from build123d import *

# Parameters (mm, degrees)
FILLET1_R           = 5
BOSS_EXTRUDE1_DEPTH = 10
CIRPATTERN1_COUNT   = 12
SKETCH3_R           = 5
CUT_EXTRUDE1_DEPTH  = 14
FILLET2_R           = 0.5
FILLET3_R           = 0.5


with BuildPart() as part:
    # Sketch1 → Revolve1 (revolve)
    with BuildSketch(Plane(origin=(0, 0, 0), x_dir=(0, 0, -1), z_dir=(1, 0, 0))):
        Polygon((-8, 0), (8, 0), (8, -25), (-11, -25), (-11, -16), (5, -16), (5, -3), (-8, -3), align=None)
    revolve(axis=Axis((0, -25, -8), (0, 0, 1)))

    # Fillet1
    fillet1_edges = [part.edges().sort_by_distance(p)[0] for p in [
        (0, -50, -8),
    ]]
    fillet(fillet1_edges, radius=FILLET1_R)

    # Sketch2 → Boss-Extrude1 (add)
    with BuildSketch(Plane(origin=(0, 0, -8), x_dir=(-1, 0, 0), z_dir=(0, 0, -1))):
        with BuildLine():
            Line((-1, -3.05572809), (1, -3.05572809))
            Line((1, -3.05572809), (1, -16.05572809))
            ThreePointArc((1, -16.05572809), (0, -16), (-1, -16.05572809))
            Line((-1, -16.05572809), (-1, -3.05572809))
        make_face()
    boss_extrude1 = extrude(amount=-BOSS_EXTRUDE1_DEPTH)

    # CirPattern1: Boss-Extrude1 ×12 about axis
    cirpattern1_axis = Axis((0, -25, 0), (0, 0, 1))
    for i in range(1, CIRPATTERN1_COUNT):
        add(boss_extrude1.rotate(cirpattern1_axis, i * 360 / CIRPATTERN1_COUNT))

    # Sketch3 → Cut-Extrude1 (cut)
    with BuildSketch(Plane.XY.offset(11)):
        with Locations((0, -25)):
            Circle(SKETCH3_R)
    extrude(amount=-CUT_EXTRUDE1_DEPTH, mode=Mode.SUBTRACT)

    # Fillet2
    fillet2_edges = [part.edges().sort_by_distance(p)[0] for p in [
        (-5, -25, 11),
        (0, -34, 11),
    ]]
    fillet(fillet2_edges, radius=FILLET2_R)

    # Fillet3
    fillet3_edges = [part.edges().sort_by_distance(p)[0] for p in [
        (0, -50, 8),
    ]]
    fillet(fillet3_edges, radius=FILLET3_R)


solid = part.part
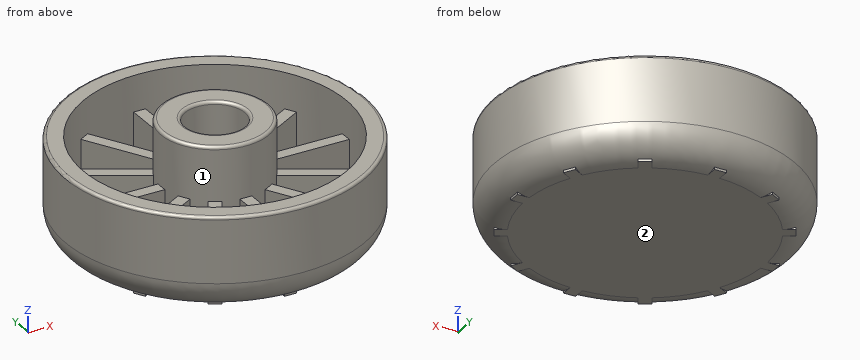
Model file for the job. Use its own axes, mm. Face numbers are marked on the shaded views. A direction names the side the tool comes from. Give positions to 0.01 mm unless a question says otherwise; leave off trailing zeros. Order: outer loops, then holes, each group sorted by start corner. A loop starts at its lowest first (then second) coordinate and runs counter-clockwise, first axis right, second up. Notation, with made-up numbers: (-25, 9) -> (-17, 9) arc R31 cw to (-17, 37) -> close; hole circle Ø3 at (-38, 19). An arc over 180 degrees is marked (long way). Use CSV: the item, a comma, the result in double quotes.
1. Band-saw the part on D-D, the plane z = -0.5. Count the separate pieces of the cut face and the enclosed holes in it, then the cut area to 3 significant figures.
Outcome:
separate pieces,"2"
enclosed holes,"2"
area,"930 mm²"
2. Drop flat-ended pins along their axis: pin 1 (3.5 mm diameter, centred on x = 18, z = -2.5, fed in from +Y); pin 2 (2 mm diameter, centred on y = -10.5, z = 0, fed in from -X); pin 3 (1.5 mm diameter, centred on x = 4.5, z = 8.5, fed in from -Y). Give the stop position or say it passes through.
Outcome:
pin 1,"y = -6"
pin 2,"x = -21.04"
pin 3,"y = -49.54"
3. Drill centre lines: line 1 along Y through (x, z) = (0, 2.75); line 2 along X through (y, z) = (-10.5, 0); line 3 along Y through (x, z) = (2, 1.5). Where is each one in solid material? Low to high. Write a range as from..to.
Outcome:
line 1,"-50..-47, -34..-30, -20..-16, -3..0"
line 2,"-20.37..-16.55, -9.53..-7.22, -1..1, 7.22..9.53, 16.55..20.37"
line 3,"-49.92..-46.91, -33.77..-29.58, -20.42..-16.23, -3.09..-0.08"
4. Band-saw the part on A-A, the plane z = 4.25. Give the cut face in (x, y), then the cut area to 3 significant figures.
Outcome:
outline,"circle Ø50 at (0, -25); circle Ø18 at (0, -25); hole circle Ø44 at (0, -25); hole circle Ø10 at (0, -25)"
area,"619 mm²"
5. 3-axis set-ups, long thin cutter, end or side, ignore diameter. For the marked faces 1 and 2: which of +Z, -Z, +X, -X, +Y, -Y reach the whole face in a straight line?
Outcome:
face 1,"+Z"
face 2,"-Z, +X, -X, +Y, -Y"
